```python
from build123d import *


with BuildPart() as part:
    # Sketch1 → Base-Revolve (revolve)
    with BuildSketch(Plane.XY):
        with BuildLine():
            Line((-140, 35), (-140, 46.5))
            ThreePointArc((-140, 46.5), (-139.707106781, 47.207106781), (-139, 47.5))
            Line((-139, 47.5), (139, 47.5))
            ThreePointArc((139, 47.5), (139.707106781, 47.207106781), (140, 46.5))
            Line((140, 46.5), (140, 35))
            Line((140, 35), (73.462610506, 35))
            Line((73.462610506, 35), (71.5, 36))
            Line((71.5, 36), (69.5, 36))
            Line((69.5, 36), (69.5, 34))
            Line((69.5, 34), (60.176326981, 34))
            ThreePointArc((60.176326981, 34), (60.002678803, 34.015192247), (59.834306837, 34.060307379))
            Line((59.834306837, 34.060307379), (50.549522195, 37.439692621))
            ThreePointArc((50.549522195, 37.439692621), (50.381150229, 37.484807753), (50.207502051, 37.5))
            Line((50.207502051, 37.5), (-50.207502051, 37.5))
            ThreePointArc((-50.207502051, 37.5), (-50.381150229, 37.484807753), (-50.549522195, 37.439692621))
            Line((-50.549522195, 37.439692621), (-59.834306837, 34.060307379))
            ThreePointArc((-59.834306837, 34.060307379), (-60.002678803, 34.015192247), (-60.176326981, 34))
            Line((-60.176326981, 34), (-69.5, 34))
            Line((-69.5, 34), (-69.5, 36))
            Line((-69.5, 36), (-71.5, 36))
            Line((-71.5, 36), (-73.462610506, 35))
            Line((-73.462610506, 35), (-140, 35))
        make_face()
    revolve(axis=Axis((-140, 0, 0), (1, 0, 0)))

    # Sketch5 → 2.5 x 30 gr reifning (revolve, cut)
    with BuildSketch(Plane.XY):
        Polygon((140, 35.866025404), (138.5, 35), (140, 35), align=None)
        Polygon((-140, 35), (-140, 35.866025404), (-138.5, 35), align=None)
    revolve(axis=Axis((0, 0, 0), (1, 0, 0)), mode=Mode.SUBTRACT)


solid = part.part
```
Model file for the job. Use its own axes, mm. A direction names the side the tool comes from. Round coordinates to 2 decimals unless told otherwise and drop trailing zeros. Write each loop counter-clockwise with the first axis right and the second up, starting at its lowest first coordinate (ties: lowest second). Pieces come first, ordered by that corner, then holes. Notation, with made-up numbers: (14.5, 50.5) -> (53.5, 50.5) arc R32 ccw to (53.5, 82.5) -> close; hole circle Ø4 at (-1, 66.5). An arc over 180 degrees is marked (long way). Answer as CSV lines item,"result".
1. Slice it at A-A, the plane x = -4. List the corners of the cut face in (y, z).
Resolved:
outline,"circle Ø95 at (0, 0); hole circle Ø75 at (0, 0)"
2. Pin check, flat tips, straight feed: pin 1 Ø8 at (x, z) = (-48, -26.5) entering from +Y; pin 2 Ø5 at (x, z) = (-8.5, 30) entering from -Y; pin 3 Ø2 at (x, y) = (99.5, 13.5) entering from -Z. Stop position of each tip, or through.
Resolved:
pin 1,"y = 41.83"
pin 2,"y = -38.73"
pin 3,"z = -45.83"
3. Drill centre lines: line 1 (Z direction, x = -71, y = 0); line 2 (Z direction, x = -83, y = -1.5); line 3 (Y direction, x = 34, z = -22.5). Where is each one in solid material? Low to high.
Resolved:
line 1,"-47.5 to -36, 36 to 47.5"
line 2,"-47.48 to -34.97, 34.97 to 47.48"
line 3,"-41.83 to -30, 30 to 41.83"
4. Tool access for faces 1 (the face through (-0.7, -4.88, 37.18)), 2 (the face through (106, -28, -21)), 3 (the face through (-106, -28, -21)), 4 (the face through (64.77, 18.28, 28.67)), 5 (the face through (-140, -24, -27)): list every direction of +Z, -Z, +X, -X, +Y, -Y with a clear straight run to the whole face (end or side of a thin tool).
Resolved:
face 1,"none"
face 2,"+X"
face 3,"-X"
face 4,"+X, -X"
face 5,"+Z, -Z, -X, +Y, -Y"
5. Slice it at B-B, the plane x = 116. List the corners of the cut face in (y, z), plus the area to 3 significant figures.
Resolved:
outline,"circle Ø95 at (0, 0); hole circle Ø70 at (0, 0)"
area,"3,240 mm²"
6. Mould opens along Y. For faces 6 (the face through (1.95, -10.3, -46.37)), 7 (the face through (-64.9, 18.28, 28.67)), 8 (the face through (-70.514, -4.686, 35.694)), 9 (the face through (140, 24, -27)) say: +Y half, -Y half, draft (parallel to the pull), parting line (faces both ways), or undercut.
Resolved:
face 6,"parting line"
face 7,"undercut"
face 8,"undercut"
face 9,"draft"
